```python
from build123d import *

# Parameters (mm, degrees)
BOSS_EXTRUDE1_DEPTH = 10
BOSS_EXTRUDE2_DEPTH = 10
BOSS_EXTRUDE3_DEPTH = 30
BOSS_EXTRUDE5_DEPTH = 20


with BuildPart() as part:
    # Sketch1 → Boss-Extrude1 (new body)
    with BuildSketch(Plane(origin=(0, 0, 0), x_dir=(1, 0, 0), z_dir=(0, 1, 0))):
        Polygon((0, 0), (35.302133222, -35.408464948), (4.552111931, -60.990415434), (-30.75002129, -25.581950485), align=None)
    extrude(amount=BOSS_EXTRUDE1_DEPTH)

    # Sketch2 → Boss-Extrude2 (add)
    with BuildSketch(Plane(origin=(0, 10, 0), x_dir=(1, 0, 0), z_dir=(0, 1, 0))):
        Polygon((-15.375010645, -12.790975243), (-30.75002129, -25.581950485), (-16.56947049, -39.685566298), (-1.259664797, -26.948837193), align=None)
    extrude(amount=BOSS_EXTRUDE2_DEPTH)

    # Sketch3 → Boss-Extrude3 (add)
    with BuildSketch(Plane(origin=(0, 0, 0), x_dir=(1, 0, 0), z_dir=(0, 1, 0))):
        Polygon((0, 0), (-15.375010645, -12.790975243), (-1.259664797, -26.948837193), (14.115345848, -14.15786195), align=None)
    extrude(amount=BOSS_EXTRUDE3_DEPTH)

    # Sketch4 → Boss-Extrude5 (add)
    with BuildSketch(Plane(origin=(0, 0, 0), x_dir=(1, 0, 0), z_dir=(0, 1, 0))):
        Polygon((14.115345848, -14.15786195), (-1.259664797, -26.948837193), (19.927122576, -48.199440191), (35.302133222, -35.408464948), align=None)
    extrude(amount=BOSS_EXTRUDE5_DEPTH)


solid = part.part
```
Design review of the part built by this model. Coordinates are the model's own, in mm. A direction names the side the tool comes from. Coordinates: 2 decimals unless noted, no trailing zeros. Order: outer loops, then holes, each group sorted by start corner. A loop starts at its lowest first (then second) coordinate and runs counter-clockwise, first axis right, second up. Notation, with made-up numbers: (-24.5, -5) - (-6.5, -5) arc R13 ccw to (-6.5, 8) - close; hole circle Ø3 at (-25, 76.5). An arc over 180 degrees is marked (long way). One line per question, with ' | ' between items.
Q1. To check wall thickness, follow line 1 along Y through (x, z) = (3, 53.5); line 2 along X through (y, z) = (19.75, 6.5); line 3 along X through (y, z) = (3.5, 20.5). State the ranges of each line that lie inside material, in increasing order.
Answer key:
line 1: y = 0 to 10 | line 2: x = -7.81 to 6.48 | line 3: x = -24.64 to 20.44
Q2. Consider section D-D, the plane x = 11.5. Give the boundary of the cut face in (y, z), then the cut area to 3 significant figures.
Answer key:
outline: (0, 11.53) - (30, 11.53) - (30, 16.33) - (20, 16.33) - (20, 39.75) - (10, 39.75) - (10, 55.21) - (0, 55.21) - close | area: 767 mm2
Q3. The part is to be moulded in two halves that separate along X. For faces 4 (the flat face through (-9.022, 14.93, 33.406)), 5 (the flat face through (17, 20, 31)), 6 (the flat face through (6.32, 24.93, 20.643)), say which applies: +X half, -X half, draft (parallel to the pull), parting line (faces both ways), or undercut.
Answer key:
face 4: undercut | face 5: draft | face 6: +X half
Q4. For faces 1 (the flat face through (9.19, 14.93, 37.43)), 2 (the flat face through (-12.852, 4.93, 43.534)), 3 (the flat face through (-8.416, 24.93, 19.771)), list the 3-axis set-ups (+Z, -Z, +X, -X, +Y, -Y) from which the entire face can be reached by the end or side of a thin tool; tool diameter is ignored.
Answer key:
face 1: +Z, +Y | face 2: +Z, -X, +Y, -Y | face 3: +Z, -X, +Y
Q5. Consider section A-A, the plane x = -7.5. Give the boundary of the cut face in (y, z), then the cut area to 3 significant figures.
Answer key:
outline: (0, 6.24) - (30, 6.24) - (30, 20.69) - (20, 20.69) - (20, 32.14) - (10, 32.14) - (10, 48.9) - (0, 48.9) - close | area: 830 mm2
Q6. Consider section B-B, the plane y = 3.25. Give the boundary of the cut face in (x, z), then the cut area to 3 significant figures.
Answer key:
outline: (-30.75, 25.58) - (0, 0) - (35.3, 35.41) - (4.55, 60.99) - close | area: 1,990 mm2
Q7. Clearance check with flat-ended pins moving along their axes: pin 1 Ø8 at (x, y) = (1, 10) entering from +Z; pin 2 Ø8 at (y, z) = (3.5, 9.5) entering from +X; pin 3 Ø3 at (y, z) = (22.5, 30.5) entering from -X; pin 4 Ø2 at (x, z) = (-1, 31.5) entering from +Y. State where each tip first meets the part, or that it passes through.
Answer key:
pin 1: stops at z = 60.99 | pin 2: stops at x = 13.46 | pin 3: passes through | pin 4: stops at y = 10
